from build123d import *

# Parameters (mm, degrees)
SKETCH2_R          = 3
CUT_EXTRUDE1_DEPTH = 18.8


with BuildPart() as part:
    # Sketch1 → Revolve1 (revolve)
    with BuildSketch(Plane.XY):
        Polygon((-17.8, 0), (-17.8, 7.5), (-8.25, 7.5), (-8.25, 9), (-3.4, 9), (-3.4, 7.5), (0, 7.5), (0, 0), align=None)
    revolve(axis=Axis((0, 0, 0), (-1, 0, 0)))

    # Sketch2 → Cut-Extrude1 (cut, through all)
    with BuildSketch(Plane.ZY.offset(17.8)):
        Circle(SKETCH2_R)
    extrude(amount=-CUT_EXTRUDE1_DEPTH, mode=Mode.SUBTRACT)


solid = part.part
Here's how the part is built. I have some questions about the finished solid (model axes, mm). A direction names the side the tool comes from. Give positions to 0.01 mm unless a question says otherwise; leave off trailing zeros. Order: outer loops, then holes, each group sorted by start corner. A loop starts at its lowest first (then second) coordinate and runs counter-clockwise, first axis right, second up. Notation, with made-up numbers: (84.5, -0.75) -> (130.5, -0.75) arc R12 ccw to (130.5, 21.25) -> close; hole circle Ø3 at (38, 80). An arc over 180 degrees is marked (long way). Use a Markdown table: item, result. Add a question column.
Item 1: Imagine slicing it at A-A on y = 0. Please give me the cut outline in (x, z), plus the area to 3 significant figures.
Item 2: I need wall thicknesses on line 1 (Y direction, x = -11, z = 0); line 2 (Y direction, x = -4.5, z = 0); line 3 (Z direction, x = -12.5, y = -0.5). Which ranges of each line are inside material? Lowest first, please.
Item 3: If we mould it in two halves opening along Z, with no side actions, what happens to faces 3 (the face through (-9, 0, -3)), 4 (the face through (-8.25, 2, -7.4)), 5 (the face through (-12.958, -7.493, -0.33))? For each: pulls with the +Z half, pulls with the -Z half, needs draft (parallel to the pull), parting line crosses it, or undercut.
Item 4: Will these pins go through, and if not, where does the flat tip stop? pin 1 (4 mm diameter, centred on y = -4.5, z = 3, fed in from +X); pin 2 (1.5 mm diameter, centred on y = -5, z = -7, fed in from +X); pin 3 (3 mm diameter, centred on x = -12, y = 5.5, fed in from +Z); pin 4 (1.5 mm diameter, centred on x = -16, z = 0, fed in from +Y).
Item 5: For faces 1 (the face through (-5.791, -1.172, -8.923)), 2 (the face through (-3.4, -2, -7.4)), which set-ups out of +Z, -Z, +X, -X, +Y, -Y let a thin tool reach every point of the face, with its end or its side?
Item 6: Imagine slicing it at D-D on y = 5.5. Please give me the cut outline in (x, z), plus the area to 3 significant figures.
Item 7: Imagine slicing it at C-C on z = -3.75. Please give me the cut outline in (x, y), plus the area to 3 significant figures.
Data:
| question | item | result |
|---|---|---|
| 1 | outline | (-17.8, -7.5) -> (-8.25, -7.5) -> (-8.25, -9) -> (-3.4, -9) -> (-3.4, -7.5) -> (0, -7.5) -> (0, -3) -> (-17.8, -3) -> close; (-17.8, 3) -> (0, 3) -> (0, 7.5) -> (-3.4, 7.5) -> (-3.4, 9) -> (-8.25, 9) -> (-8.25, 7.5) -> (-17.8, 7.5) -> close |
| 1 | area | 175 mm² |
| 2 | line 1 | y = -7.5 to -3, 3 to 7.5 |
| 2 | line 2 | y = -9 to -3, 3 to 9 |
| 2 | line 3 | z = -7.48 to -2.96, 2.96 to 7.48 |
| 3 | face 3 | undercut |
| 3 | face 4 | needs draft |
| 3 | face 5 | parting line crosses it |
| 4 | pin 1 | stops at x = 0 |
| 4 | pin 2 | stops at x = -3.4 |
| 4 | pin 3 | stops at z = 6.34 |
| 4 | pin 4 | stops at y = 7.5 |
| 5 | face 1 | +X, -X |
| 5 | face 2 | +X |
| 6 | outline | (-17.8, -5.1) -> (-8.25, -5.1) -> (-8.25, -7.12) -> (-3.4, -7.12) -> (-3.4, -5.1) -> (0, -5.1) -> (0, 5.1) -> (-3.4, 5.1) -> (-3.4, 7.12) -> (-8.25, 7.12) -> (-8.25, 5.1) -> (-17.8, 5.1) -> close |
| 6 | area | 201 mm² |
| 7 | outline | (-17.8, -6.5) -> (-8.25, -6.5) -> (-8.25, -8.18) -> (-3.4, -8.18) -> (-3.4, -6.5) -> (0, -6.5) -> (0, 6.5) -> (-3.4, 6.5) -> (-3.4, 8.18) -> (-8.25, 8.18) -> (-8.25, 6.5) -> (-17.8, 6.5) -> close |
| 7 | area | 248 mm² |
